Could you check a few things on this drawing? It's one solid part, dimensions in mm from its lowest x, y, z. Round coordinates to 2 decimals unless told otherwise and drop trailing zeros. Loops run counter-clockwise (first coordinate to the right, second up) from the corner with the lowest first, then second, coordinate; pieces in that order, holes last. Notation, with made-up numbers: M 34.25,71 L 68.25,71 A12 ccw 68.25,91 Z; hole C 54.25,89.25 d9. An arc over 180 degrees is marked long. Write each question's results on one line, items separated by ' | '. Start each with the question number.
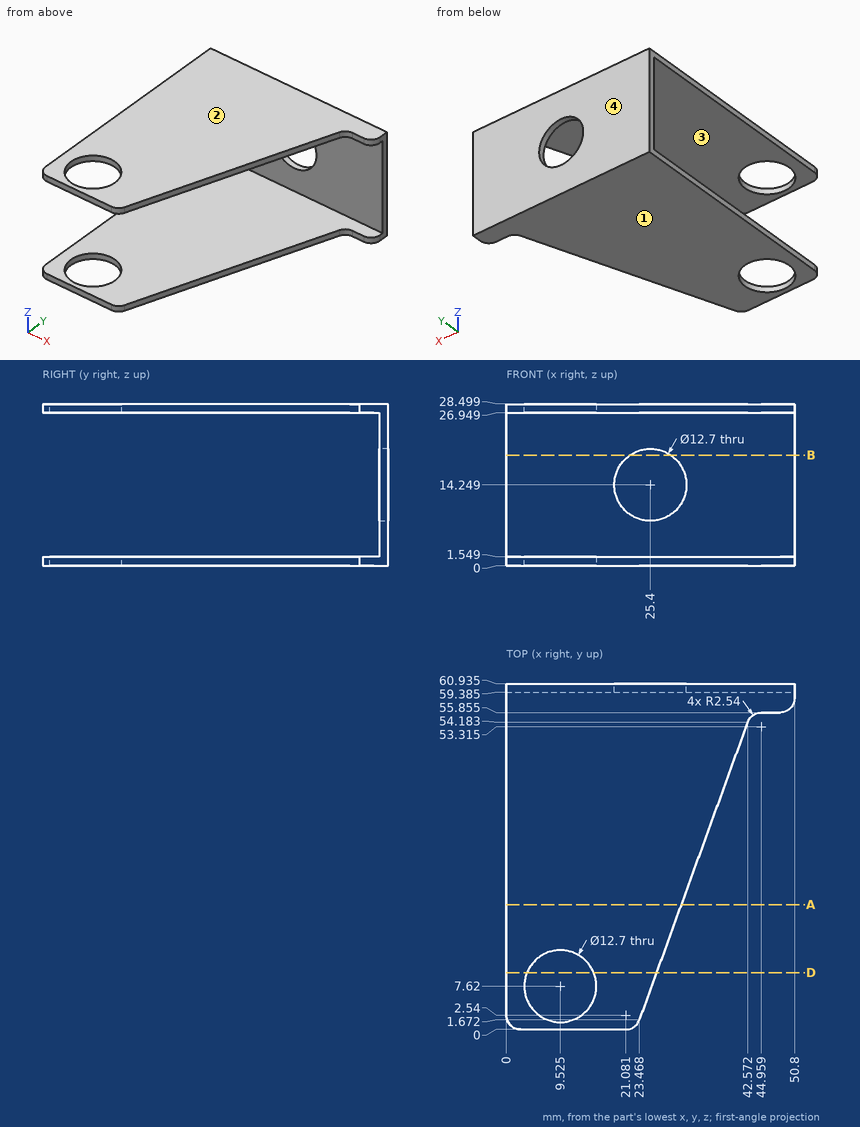
1. I need wall thicknesses on line 1 along Z through (x, y) = (23.5, 46); line 2 along Y through (x, z) = (21.5, 3.25) (1 decimal). Which ranges of each line are inside material? Lowest first, please.
2. If we mould it in two halves opening along Z, with no side actions, what happens to the marked faces 1, 2, 3 and 4? For each: released by +Z, released by -Z, zero draft, split by the parting line, or undercut.
3. For pin 1 (1.7 mm diameter, centred on x = 47.5, z = 28, fed in from -Y) (1 decimal); pin 2 (1.5 mm diameter, centred on x = 32, z = 11.5, fed in from -Y) (1 decimal), each with a flat end and sliding along its axis, tell me the tip position at first contact or that it passes through.
4. I want a section at B-B on z = 19.5. List the corners of the cut face in (x, y) for me (1 decimal).
5. I want a section at A-A on y = 22. List the corners of the cut face in (x, z) for me.
6. I want a section at D-D on y = 10. List the corners of the cut face in (x, z) for me.
Outcome:
1) line 1: 0 to 1.55, 26.95 to 28.5 | line 2: 59.4 to 60.9
2) face 1: released by -Z | face 2: released by +Z | face 3: undercut | face 4: zero draft
3) pin 1: y = 55.9 | pin 2: y = 59.4
4) outline: M 0,59.4 L 21.8,59.4 L 21.8,60.9 L 0,60.9 Z; M 29,59.4 L 50.8,59.4 L 50.8,60.9 L 29,60.9 Z
5) outline: M 0,0 L 30.86,0 L 30.86,1.55 L 0,1.55 Z; M 0,26.95 L 30.86,26.95 L 30.86,28.5 L 0,28.5 Z
6) outline: M 0,0 L 3.64,0 L 3.64,1.55 L 0,1.55 Z; M 0,26.95 L 3.64,26.95 L 3.64,28.5 L 0,28.5 Z; M 15.41,0 L 26.5,0 L 26.5,1.55 L 15.41,1.55 Z; M 15.41,26.95 L 26.5,26.95 L 26.5,28.5 L 15.41,28.5 Z
